Study the drawing (mm; zero at the part's minimum x, y, z) and answer. Coordinates: 2 decimals unless noted, no trailing zeros. Loops run counter-clockwise (first coordinate to the right, second up) from the corner with the lowest first, then second, coordinate; pieces in that order, holes last. Notation, with made-up numbers: (29, 18) - (59, 18) arc R29 cw to (59, 54) - close; hole circle Ø9 at (6, -34). An arc over 180 degrees is marked (long way). Use one line per item in the form item = value. Start each with the question number.
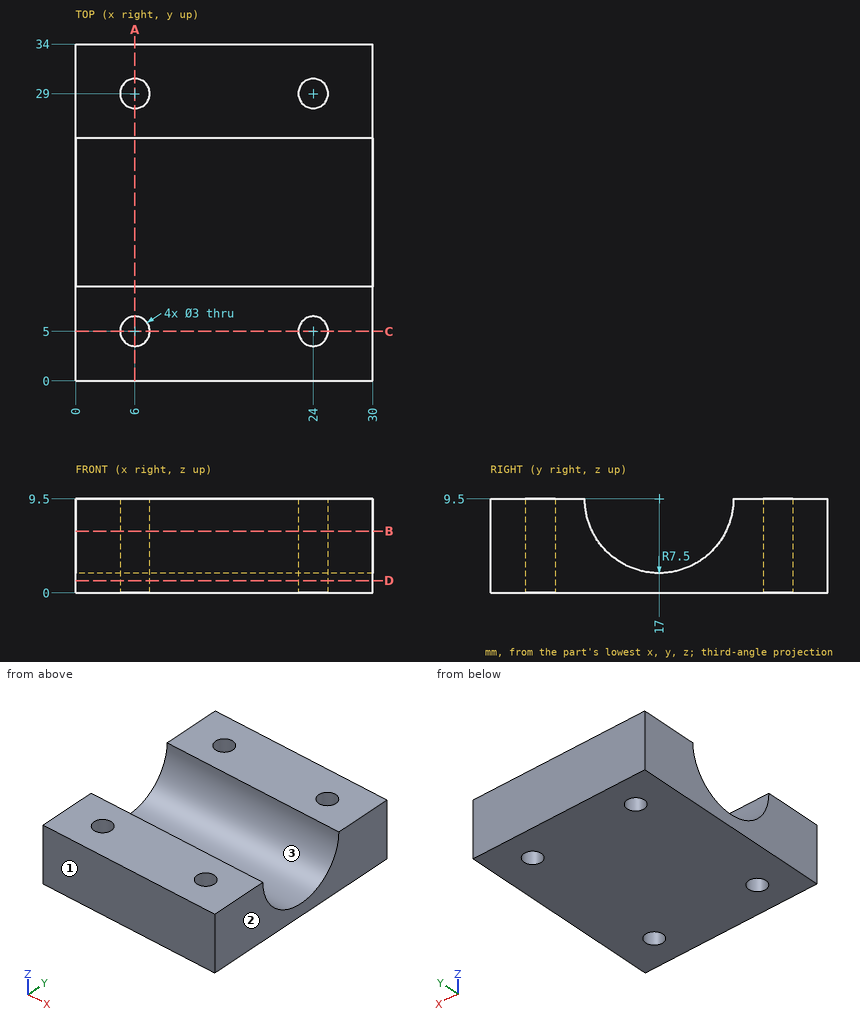
(1) Determine the mould class of the marked faces 1, 2 and 3 for opening direction Y: +Y half, -Y half, draft (parallel to the pull), parting line (faces both ways), or undercut.
(2) Find the intervals of material crossed by probe 1 along Y at (x, z) = (23.25, 1.5); probe 2 along Y at (x, z) = (6, 2.75); probe 3 along Y at (x, z) = (6, 5.25), in increasing order. Write a range as from..to.
(3) A cutting plane is placed at A-A (x = 6). Determine the outline of the cut face in (y, z), then the cut area to 3 significant figures.
(4) A cutting plane is placed at C-C (y = 5). Determine the outline of the cut face in (x, z).
(5) This flat-tipped pin is pushed along its axis until it touches: pin 1 Ø1.5 at (x, y) = (24, 16) entering from +Z. Where does it stop, or does it pass through?
(6) A cutting plane is placed at B-B (z = 6.25). Determine the outline of the cut face in (x, y).
(7) A cutting plane is placed at D-D (z = 1.25). Determine the outline of the cut face in (x, y).
Evaluation:
q1.face_1 = -Y half
q1.face_2 = draft
q1.face_3 = undercut
q2.probe_1 = 0..3.7, 6.3..27.7, 30.3..34
q2.probe_2 = 0..3.5, 6.5..13.73, 20.27..27.5, 30.5..34
q2.probe_3 = 0..3.5, 6.5..10.82, 23.18..27.5, 30.5..34
q3.outline = (0, 0) - (3.5, 0) - (3.5, 9.5) - (0, 9.5) - close; (6.5, 0) - (27.5, 0) - (27.5, 9.5) - (24.5, 9.5) arc R7.5 cw to (9.5, 9.5) - (6.5, 9.5) - close; (30.5, 0) - (34, 0) - (34, 9.5) - (30.5, 9.5) - close
q3.area = 178 mm^2
q4.outline = (0, 0) - (4.5, 0) - (4.5, 9.5) - (0, 9.5) - close; (7.5, 0) - (22.5, 0) - (22.5, 9.5) - (7.5, 9.5) - close; (25.5, 0) - (30, 0) - (30, 9.5) - (25.5, 9.5) - close
q5.pin_1 = 2.21
q6.outline = (0, 0) - (30, 0) - (30, 10.24) - (0, 10.24) - close; (0, 23.76) - (30, 23.76) - (30, 34) - (0, 34) - close; hole circle Ø3 at (6, 5); hole circle Ø3 at (6, 29); hole circle Ø3 at (24, 5); hole circle Ø3 at (24, 29)
q7.outline = (0, 0) - (30, 0) - (30, 34) - (0, 34) - close; hole circle Ø3 at (6, 5); hole circle Ø3 at (6, 29); hole circle Ø3 at (24, 5); hole circle Ø3 at (24, 29)
